Build history of the part. All positions in model axes, mm. Round coordinates to 2 decimals unless told otherwise and drop trailing zeros. Use a Markdown table: item, result. Add a question column.
Item 1: Slice it at A-A, the plane z = -242.5. State how many separate pieces and enclosed holes the cut face has, plus the area to 3 significant figures.
Item 2: Probe L1, parallel to X at y = 8, z = -60.5; L2, parallel to Y at x = 0, z = -146.5; L3, parallel to X at y = -6, z = -289.5. List the from-to ranges inside material, lowest first.
Item 3: Pin check, flat tips, straight feed: pin 1 (4 mm diameter, centred on x = 0.5, z = -161.5, fed in from -Y); pin 2 (3 mm diameter, centred on x = -0.5, z = -130, fed in from +Y); pin 3 (1 mm diameter, centred on x = -7.5, y = 3.5, fed in from -Z). Stop position of each tip, or through.
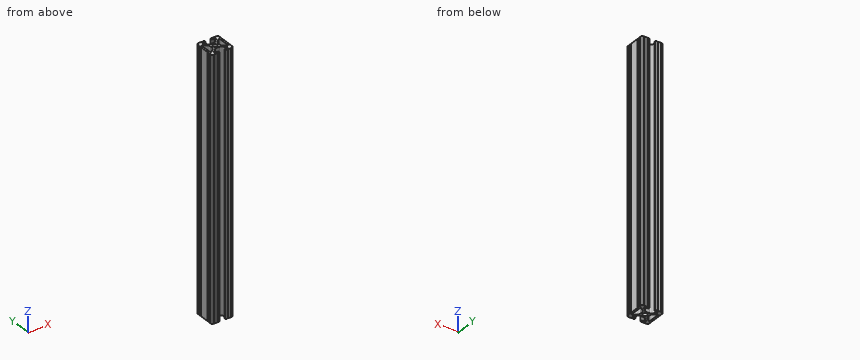
Autodesk Inventor part; units mm, degrees
ref_plane "YZ Plane" through (0, 0, 0) normal (1, 0, 0) x (0, 1, 0)
ref_plane "XZ Plane" through (0, 0, 0) normal (0, 1, 0) x (-1, 0, 0)
ref_plane "XY Plane" through (0, 0, 0) normal (0, 0, 1) x (1, 0, 0)
sketch "Sketch1" plane through (0, 0, 0) normal (0, 0, 1) x (1, 0, 0)
  arc A0 (5.4405, 3.6206) -> (4.5085, 1.3735) centre (7.6835, 1.3735) ccw
  line L0 (9.0008, 7.1744) -> (5.4405, 3.6206)
  arc A1 (10.4902, 6.5567) -> (9.0008, 7.1744) centre (9.6174, 6.5567) ccw
  line L1 (10.4902, -6.5567) -> (10.4902, 6.5567)
  arc A2 (9.0008, -7.1744) -> (10.4902, -6.5567) centre (9.6174, -6.5567) ccw
  line L2 (5.4405, -3.6206) -> (9.0008, -7.1744)
  arc A3 (4.5085, -1.3735) -> (5.4405, -3.6206) centre (7.6835, -1.3735) ccw
  line L3 (4.5085, 1.3735) -> (4.5085, -1.3735)
  circle A4 centre (0, 0) radius 2.6035
  arc A5 (-9.0008, 7.1744) -> (-10.4902, 6.5567) centre (-9.6174, 6.5567) ccw
  line L4 (-5.4405, 3.6206) -> (-9.0008, 7.1744)
  arc A6 (-4.5085, 1.3735) -> (-5.4405, 3.6206) centre (-7.6835, 1.3735) ccw
  line L5 (-4.5085, -1.3735) -> (-4.5085, 1.3735)
  arc A7 (-5.4405, -3.6206) -> (-4.5085, -1.3735) centre (-7.6835, -1.3735) ccw
  line L6 (-9.0008, -7.1744) -> (-5.4405, -3.6206)
  arc A8 (-10.4902, -6.5567) -> (-9.0008, -7.1744) centre (-9.6174, -6.5567) ccw
  line L7 (-10.4902, 6.5567) -> (-10.4902, -6.5567)
  arc A9 (-7.3891, -8.6879) -> (-6.6435, -10.4902) centre (-6.6435, -9.4348) ccw
  line L8 (-7.3891, -8.6879) -> (-4.1189, -5.4237)
  arc A10 (-1.8759, -4.4958) -> (-4.1189, -5.4237) centre (-1.8759, -7.6708) ccw
  line L9 (-1.8759, -4.4958) -> (1.8759, -4.4958)
  arc A11 (4.1189, -5.4237) -> (1.8759, -4.4958) centre (1.8759, -7.6708) ccw
  line L10 (4.1189, -5.4237) -> (7.3891, -8.6879)
  arc A12 (6.6435, -10.4902) -> (7.3891, -8.6879) centre (6.6435, -9.4348) ccw
  line L11 (6.6435, -10.4902) -> (4.2875, -10.4902)
  arc A13 (4.2875, -10.4902) -> (3.2385, -11.5392) centre (4.2875, -11.5392) ccw
  line L12 (3.2385, -11.5392) -> (3.2385, -11.651)
  arc A14 (3.2385, -11.651) -> (4.2875, -12.7) centre (4.2875, -11.651) ccw
  line L13 (4.2875, -12.7) -> (5.3171, -12.7)
  arc A15 (6.3331, -12.7) -> (5.3171, -12.7) centre (5.8251, -12.7) ccw
  line L14 (6.3331, -12.7) -> (9.5504, -12.7)
  arc A16 (10.5664, -12.6998) -> (9.5504, -12.7) centre (10.0584, -12.7) ccw
  arc A17 (10.5664, -12.6998) -> (12.6998, -10.5664) centre (10.5918, -10.5918) ccw
  arc A18 (12.7, -9.5504) -> (12.6998, -10.5664) centre (12.7, -10.0584) ccw
  line L15 (12.7, -9.5504) -> (12.7, -6.3331)
  arc A19 (12.7, -5.3171) -> (12.7, -6.3331) centre (12.7, -5.8251) ccw
  line L16 (12.7, -5.3171) -> (12.7, 5.3171)
  arc A20 (12.7, 6.3331) -> (12.7, 5.3171) centre (12.7, 5.8251) ccw
  line L17 (12.7, 6.3331) -> (12.7, 9.5504)
  arc A21 (12.6998, 10.5664) -> (12.7, 9.5504) centre (12.7, 10.0584) ccw
  arc A22 (12.6998, 10.5664) -> (10.5664, 12.6998) centre (10.5918, 10.5918) ccw
  arc A23 (9.5504, 12.7) -> (10.5664, 12.6998) centre (10.0584, 12.7) ccw
  line L18 (9.5504, 12.7) -> (6.3331, 12.7)
  arc A24 (5.3171, 12.7) -> (6.3331, 12.7) centre (5.8251, 12.7) ccw
  line L19 (5.3171, 12.7) -> (4.2875, 12.7)
  arc A25 (4.2875, 12.7) -> (3.2385, 11.651) centre (4.2875, 11.651) ccw
  line L20 (3.2385, 11.651) -> (3.2385, 11.5392)
  arc A26 (3.2385, 11.5392) -> (4.2875, 10.4902) centre (4.2875, 11.5392) ccw
  line L21 (4.2875, 10.4902) -> (6.6858, 10.4902)
  arc A27 (7.419, 8.7178) -> (6.6858, 10.4902) centre (6.6858, 9.4523) ccw
  line L22 (7.419, 8.7178) -> (4.1189, 5.4237)
  arc A28 (1.8759, 4.4958) -> (4.1189, 5.4237) centre (1.8759, 7.6708) ccw
  line L23 (1.8759, 4.4958) -> (-1.8759, 4.4958)
  arc A29 (-4.1189, 5.4237) -> (-1.8759, 4.4958) centre (-1.8759, 7.6708) ccw
  line L24 (-4.1189, 5.4237) -> (-7.419, 8.7178)
  arc A30 (-6.6858, 10.4902) -> (-7.419, 8.7178) centre (-6.6858, 9.4523) ccw
  line L25 (-6.6858, 10.4902) -> (-4.2875, 10.4902)
  arc A31 (-4.2875, 10.4902) -> (-3.2385, 11.5392) centre (-4.2875, 11.5392) ccw
  line L26 (-3.2385, 11.5392) -> (-3.2385, 11.651)
  arc A32 (-3.2385, 11.651) -> (-4.2875, 12.7) centre (-4.2875, 11.651) ccw
  line L27 (-4.2875, 12.7) -> (-5.3171, 12.7)
  arc A33 (-6.3331, 12.7) -> (-5.3171, 12.7) centre (-5.8251, 12.7) ccw
  line L28 (-6.3331, 12.7) -> (-9.5504, 12.7)
  arc A34 (-10.5664, 12.6998) -> (-9.5504, 12.7) centre (-10.0584, 12.7) ccw
  arc A35 (-10.5664, 12.6998) -> (-12.6998, 10.5664) centre (-10.5918, 10.5918) ccw
  arc A36 (-12.7, 9.5504) -> (-12.6998, 10.5664) centre (-12.7, 10.0584) ccw
  line L29 (-12.7, 9.5504) -> (-12.7, 6.3331)
  arc A37 (-12.7, 5.3171) -> (-12.7, 6.3331) centre (-12.7, 5.8251) ccw
  line L30 (-12.7, 5.3171) -> (-12.7, -5.3171)
  arc A38 (-12.7, -6.3331) -> (-12.7, -5.3171) centre (-12.7, -5.8251) ccw
  line L31 (-12.7, -6.3331) -> (-12.7, -9.5504)
  arc A39 (-12.6998, -10.5664) -> (-12.7, -9.5504) centre (-12.7, -10.0584) ccw
  arc A40 (-12.6998, -10.5664) -> (-10.5664, -12.6998) centre (-10.5918, -10.5918) ccw
  arc A41 (-9.5504, -12.7) -> (-10.5664, -12.6998) centre (-10.0584, -12.7) ccw
  line L32 (-9.5504, -12.7) -> (-6.3331, -12.7)
  arc A42 (-5.3171, -12.7) -> (-6.3331, -12.7) centre (-5.8251, -12.7) ccw
  line L33 (-5.3171, -12.7) -> (-4.2875, -12.7)
  arc A43 (-4.2875, -12.7) -> (-3.2385, -11.651) centre (-4.2875, -11.651) ccw
  line L34 (-3.2385, -11.651) -> (-3.2385, -11.5392)
  arc A44 (-3.2385, -11.5392) -> (-4.2875, -10.4902) centre (-4.2875, -11.5392) ccw
  line L35 (-4.2875, -10.4902) -> (-6.6435, -10.4902)
extrude "Extrusion1" add sketch "Sketch1" against normal blind 304.8
properties part number "1004"
Check sheet entries:
| question | item | result |
|---|---|---|
| 1 | separate pieces | 1 |
| 1 | enclosed holes | 3 |
| 1 | area | 310 mm2 |
| 2 | L1 | -12.7 to -6.7, 6.7 to 12.7 |
| 2 | L2 | -4.5 to -2.6, 2.6 to 4.5 |
| 2 | L3 | -12.22 to -10.49, -7.82 to -4.7, 4.7 to 7.82, 10.49 to 12.22 |
| 3 | pin 1 | y = -4.56 |
| 3 | pin 2 | y = 4.5 |
| 3 | pin 3 | through |
